```python
from build123d import *

# Parameters (mm, degrees)
SKETCH_1_W          = 8
SKETCH_1_H          = 16
EXTRUDE_1_DEPTH     = 10
SKETCH_2_R          = 0.852
CUT_EXTRUDE_1_DEPTH = 20.287301522
SKETCH_3_W          = 11.235534132
SKETCH_3_H          = 3.949082568
CUT_EXTRUDE_2_DEPTH = 7
CHAMFER_1_SIZE      = 2


with BuildPart() as part:
    # Эскиз1 → Вытянуть1 (new body)
    with BuildSketch(Plane(origin=(0, 0, 0), x_dir=(1, 0, 0), z_dir=(0, 1, 0))):
        Rectangle(SKETCH_1_W, SKETCH_1_H)
    extrude(amount=EXTRUDE_1_DEPTH)

    # Эскиз2 → Вырез-Вытянуть1 (cut, through all)
    with BuildSketch(Plane.XY.offset(8)):
        with Locations((0, 6.986387237)):
            Circle(SKETCH_2_R)
    extrude(amount=-CUT_EXTRUDE_1_DEPTH, mode=Mode.SUBTRACT)

    # Эскиз3 → Вырез-Вытянуть2 (cut)
    with BuildSketch(Plane(origin=(0, 10, 0), x_dir=(1, 0, 0), z_dir=(0, 1, 0))):
        Rectangle(SKETCH_3_W, SKETCH_3_H)
    extrude(amount=-CUT_EXTRUDE_2_DEPTH, mode=Mode.SUBTRACT)

    # Фаска1
    chamfer_1_edges = [part.edges().sort_by_distance(p)[0] for p in [
        (-4, 10, -4.987270642),
        (4, 10, -4.987270642),
        (-4, 10, 4.987270642),
        (4, 10, 4.987270642),
    ]]
    chamfer(chamfer_1_edges, length=CHAMFER_1_SIZE)


solid = part.part
```
The model under review builds one solid part; all positions refer to its coordinate system, in mm. A direction names the side the tool comes from. Round coordinates to 2 decimals unless told otherwise and drop trailing zeros. Order: outer loops, then holes, each group sorted by start corner. A loop starts at its lowest first (then second) coordinate and runs counter-clockwise, first axis right, second up. Notation, with made-up numbers: (38.5, -17) -> (55.5, -17) arc R25 ccw to (55.5, 17) -> close; hole circle Ø5 at (32.5, 80). An arc over 180 degrees is marked (long way). One line per item, written item: value. Start each with the question number.
Q1. Wall thickness on line 1 (Z direction, x = -2.75, y = 3.5); line 2 (Y direction, x = 0, z = -6.5); line 3 (X direction, y = 7, z = -3.5): over which ranges is each line inside the solid? List them lowest first.
Q2. Take a section at A-A (y = 9.25). Write out the cut boundary in (x, z), and give its area (3 significant figures).
Q3. Clearance check with a flat-ended pin moving along its axis: pin 1 Ø1.4 at (x, y) = (0, 6.99) entering from +Z. State where the tip first meets the part, or that it passes through.
Q4. Take a section at D-D (y = 6.5). Write out the cut boundary in (x, z).
Q5. Machinability: for faces 1 (the face through (-3, 9, -5)), 2 (the face through (-0.1, 5.8, -1.975)), which of the approach directions +Z, -Z, +X, -X, +Y, -Y give a long, thin tool a straight path to every point of the face, cutting with its end or side? Answer none if there is none.
Q6. Mouldability with a two-part tool opening along X and no side actions: class faces 3 (the face through (-0.185, 6.155, -4.945)), 4 (the face through (-3, 9, 5)), 5 (the face through (-0.185, 6.155, 5.029)), 6 (the face through (0, 10, -5)) as released by +X, released by -X, zero draft, split by the parting line, or undercut.
Q7. Take a section at B-B (x = 0). Write out the cut boundary in (y, z), and give its area (3 significant figures).
Q8. Take a section at C-C (x = 1.75). Write out the cut boundary in (y, z), and give its area (3 significant figures).
Reported:
1. line 1: z = -8 to -1.97, 1.97 to 8
1. line 2: y = 0 to 6.13, 7.84 to 10
1. line 3: x = -4 to -0.85, 0.85 to 4
2. outline: (-2.75, -8) -> (2.75, -8) -> (2.75, -1.97) -> (-2.75, -1.97) -> close; (-2.75, 1.97) -> (2.75, 1.97) -> (2.75, 8) -> (-2.75, 8) -> close
2. area: 66.3 mm2
3. pin 1: passes through
4. outline: (-4, -8) -> (-0.7, -8) -> (-0.7, -1.97) -> (-4, -1.97) -> close; (-4, 1.97) -> (-0.7, 1.97) -> (-0.7, 8) -> (-4, 8) -> close; (0.7, -8) -> (4, -8) -> (4, -1.97) -> (0.7, -1.97) -> close; (0.7, 1.97) -> (4, 1.97) -> (4, 8) -> (0.7, 8) -> close
5. face 1: +Z, -Z, -X, +Y
5. face 2: +X, -X, +Y
6. face 3: undercut
6. face 4: released by -X
6. face 5: undercut
6. face 6: zero draft
7. outline: (0, -8) -> (6.13, -8) -> (6.13, -1.97) -> (3, -1.97) -> (3, 1.97) -> (6.13, 1.97) -> (6.13, 8) -> (0, 8) -> close; (7.84, -8) -> (10, -8) -> (10, -1.97) -> (7.84, -1.97) -> close; (7.84, 1.97) -> (10, 1.97) -> (10, 8) -> (7.84, 8) -> close
7. area: 112 mm2
8. outline: (0, -8) -> (10, -8) -> (10, -1.97) -> (3, -1.97) -> (3, 1.97) -> (10, 1.97) -> (10, 8) -> (0, 8) -> close
8. area: 132 mm2
